Part print with two shaded views. Sizes in mm from the minimum x, y, z corner. A direction names the side the tool comes from. Round coordinates to 2 decimals unless told otherwise and drop trailing zeros. Write each loop counter-clockwise with the first axis right and the second up, starting at its lowest first coordinate (ties: lowest second). Pieces come first, ordered by that corner, then holes. Notation, with made-up numbers: M -23.5,16.25 L 31.5,16.25 A9 cw 31.5,21.25 Z; hole C 82,-31 d6. An arc over 180 degrees is marked long. Use one line per item in the form item = value. Start each with the question number.
Item 1: Which spindle directions (+Z, -Z, +X, -X, +Y, -Y) get a long thin tool onto all of the face, cutting with end or side? Do the marked faces 4 and 5. Say none if no direction does.
Item 2: Cut at B-B, the plane z = 52. Give the cut face in (x, y) (1 decimal), then the cut area to 3 significant figures.
Item 3: Mould opens along X. For the marked faces 1, 2 and 3 say: +X half, -X half, draft (parallel to the pull), parting line (faces both ways), or undercut.
Item 4: Flat gauge pin, fed straight in: pin 1 Ø4 at (x, z) = (12.7, 12.7) entering from +Y. Where does the tip first touch, or does it go through?
Item 5: Cut at A-A, the plane x = 12.7. State how many separate pieces and enclosed holes the cut face has.
Item 6: Probe L1, parallel to Z at x = 12.7, y = 24.7; L2, parallel to Y at x = 21.75, z = 64.5 (1 decimal). List the from-to ranges inside material, lowest first.
Item 7: Cut at C-C, the plane y = 15. Give the cut face in (x, z) (1 decimal).
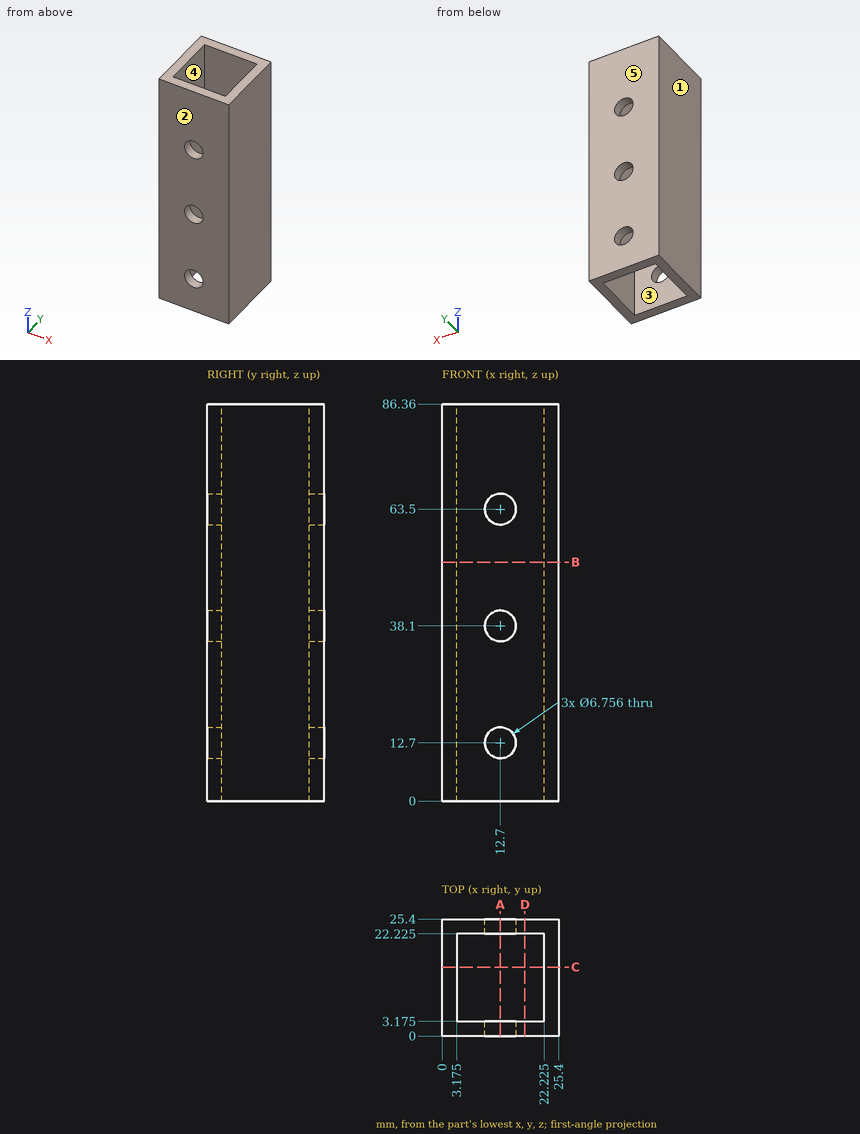
Model answer:
q1.face_4 = +Z, -Z
q1.face_5 = +Z, -Z, +X, -X, +Y
q2.outline = M 0,0 L 25.4,0 L 25.4,25.4 L 0,25.4 Z; hole M 3.2,3.2 L 22.2,3.2 L 22.2,22.2 L 3.2,22.2 Z
q2.area = 282 mm²
q3.face_1 = -X half
q3.face_2 = draft
q3.face_3 = undercut
q4.pin_1 = through
q5.separate_pieces = 8
q5.enclosed_holes = 0
q6.L1 = 0 to 9.32, 16.08 to 34.72, 41.48 to 60.12, 66.88 to 86.36
q6.L2 = 0 to 3.2, 22.2 to 25.4
q7.outline = M 0,0 L 3.2,0 L 3.2,86.4 L 0,86.4 Z; M 22.2,0 L 25.4,0 L 25.4,86.4 L 22.2,86.4 Z
